Build history of the part. All positions in model axes, mm. A direction names the side the tool comes from. Give positions to 0.01 mm unless a question says otherwise; leave off trailing zeros. Loops run counter-clockwise (first coordinate to the right, second up) from the corner with the lowest first, then second, coordinate; pieces in that order, holes last. Notation, with made-up numbers: M 65,-39 L 87,-39 A11 cw 87,-31 Z; hole C 8,-1.5 d1. An arc over 180 degrees is marked long. Answer as a JSON object with one key per item and string values. Group by question number.
1. Slice it at A-A (y = 0). List the corners of the cut face in (x, z), then the cut area to 3 significant figures.
2. Drill centre lines: line 1 along Z through (x, y) = (0, -3.05); line 2 along Y through (x, z) = (9.5, -26); line 3 along X through (y, z) = (-0.25, -3.5). Where is each one in solid material? Low to high. Write a range as [from, to].
3. 3-axis set-ups, long thin cutter, end or side, ignore diameter. For faces 1 (the face through (-0.65, -3.91, 22.07)), 2 (the face through (23.938, -2.584, -1.984)), 3 (the face through (-0.521, 1.028, -28.966)): which of +Z, -Z, +X, -X, +Y, -Y reach the whole face in a straight line?
4. Mould opens along Z. For faces 4 (the face through (-20, 3, 0)), 5 (the face through (-25.9, -3.91, 2.86)), 6 (the face through (-28.2, 1, 2.4)) say: released by +Z, released by -Z, zero draft, split by the parting line, or undercut.
5. Drop flat-ended pins along their axis: pin 1 Ø2.5 at (x, z) = (0.5, -23.5) entering from +Y; pin 2 Ø1 at (y, z) = (0, 6) entering from +X; pin 3 Ø3 at (x, y) = (15, -0.5) entering from -Z. Give the stop position or say it passes through.
from build123d import *

# Parameters (mm, degrees)
SKETCH1_R                      = 32
SKETCH1_R_2                    = 18
BOSS_EXTRUDE1_DEPTH            = 3
CBORE_FOR_M4_SHCS1_D           = 4.5
CBORE_FOR_M4_SHCS1_CBORE_D     = 8
CBORE_FOR_M4_SHCS1_CBORE_DEPTH = 4
CHAMFER1_SIZE                  = 1
BOSS_EXTRUDE2_START            = 2
SKETCH4_R                      = 3
SKETCH4_R_2                    = 2.25
BOSS_EXTRUDE2_DEPTH            = 2
CHAMFER2_SIZE                  = 0.2
CIRPATTERN1_COUNT              = 4
CHAMFER2_OF_CIRPATTERN1_SIZE   = 0.2


with BuildPart() as part:
    # Sketch1 → Boss-Extrude1 (new, symmetric)
    with BuildSketch(Plane(origin=(0, 0, 0), x_dir=(1, 0, 0), z_dir=(0, 1, 0))):
        with Locations(Location((0, 0, 0), (0, 0, 270))):
            Circle(SKETCH1_R)
        with Locations(Location((0, 0, 0), (0, 0, 270))):
            Circle(SKETCH1_R_2, mode=Mode.SUBTRACT)
    extrude(amount=BOSS_EXTRUDE1_DEPTH, both=True)

    # CBORE for M4 SHCS1 (through all)
    with Locations(Plane(origin=(0, 3, 0), x_dir=(1, 0, 0), z_dir=(0, 1, 0))):
        with Locations((-25, 0), (0, 25), (25, 0), (0, -25)):
            CounterBoreHole(CBORE_FOR_M4_SHCS1_D / 2, CBORE_FOR_M4_SHCS1_CBORE_D / 2, CBORE_FOR_M4_SHCS1_CBORE_DEPTH)

    # Chamfer1
    chamfer1_edges = [part.edges().sort_by_distance(p)[0] for p in [
        (0, -3, -32),
        (0, 3, -32),
        (0, -3, -18),
        (0, 3, -18),
    ]]
    chamfer(chamfer1_edges, length=CHAMFER1_SIZE)

    # Sketch4 → Boss-Extrude2 (add)
    with BuildSketch(Plane.XZ.offset(3).offset(BOSS_EXTRUDE2_START)):
        with Locations(Location((-25, 0, 0), (0, 0, 90))):
            Circle(SKETCH4_R)
        with Locations(Location((-25, 0, 0), (0, 0, 90))):
            Circle(SKETCH4_R_2, mode=Mode.SUBTRACT)
    boss_extrude2 = extrude(amount=-BOSS_EXTRUDE2_DEPTH)

    # Chamfer2
    chamfer2_edges = [part.edges().sort_by_distance(p)[0] for p in [
        (-25, -5, -3),
    ]]
    chamfer(chamfer2_edges, length=CHAMFER2_SIZE)

    # CirPattern1: Boss-Extrude2 ×4 about axis
    cirpattern1_axis = Axis((0, 0, 0), (0, 1, 0))
    for i in range(1, CIRPATTERN1_COUNT):
        add(boss_extrude2.rotate(cirpattern1_axis, i * 360 / CIRPATTERN1_COUNT))

    # Chamfer2 of CirPattern1
    chamfer2_of_cirpattern1_edges = [part.edges().sort_by_distance(p)[0] for p in [
        (-3, -5, 25),
        (25, -5, 3),
        (3, -5, -25),
    ]]
    chamfer(chamfer2_of_cirpattern1_edges, length=CHAMFER2_OF_CIRPATTERN1_SIZE)


solid = part.part
Established:
{
 "1": {"outline": "C 0,0 d64; hole C -25,0 d8; hole C 0,0 d36; hole C 0,-25 d8; hole C 0,25 d8; hole C 25,0 d8", "area": "2,000 mm^2"},
 "2": {"line 1": "z = [-28, -27.25], [-22.75, -22], [22, 22.75], [27.25, 28]", "line 2": "y = [-3, 3]", "line 3": "x = [-31.81, -26.94], [-23.06, -17.66], [17.66, 23.06], [26.94, 31.81]"},
 "3": {"face 1": "-Y", "face 2": "+Y, -Y", "face 3": "+Y"},
 "4": {"face 4": "zero draft", "face 5": "split by the parting line", "face 6": "undercut"},
 "5": {"pin 1": "stops at y = -1", "pin 2": "stops at x = 31.52", "pin 3": "stops at z = -29.01"}
}
